```python
from build123d import *

# Parameters (mm, degrees)
F0_R     = 2.725
F1_DEPTH = 10
F2_R     = 1.75
F3_DEPTH = 12.5
F4_R     = 1.8
F4_R_2   = 1.75
F5_DEPTH = 1
F6_R     = 1.75
F7_DEPTH = 4
F9_R     = 1.75


# Not quite as in the source:
# - a fillet or chamfer that OpenCascade refuses, or shapes differently, is made with other operations: its cross-section is extruded or revolved along the edge and cut away or added


with BuildPart() as f1:
    # F0 (on Top) → F1 (new body)
    with BuildSketch(Plane.XY):
        Circle(F0_R)
    extrude(amount=F1_DEPTH)

    # F2 (on face) → F3 (join)
    with BuildSketch(Plane.XY.offset(10)):
        Circle(F2_R)
    extrude(amount=F3_DEPTH)

    # F4 (on face) → F5 (join)
    with BuildSketch(Plane.XY.offset(22.5)):
        Circle(F4_R)
        Circle(F4_R_2, mode=Mode.SUBTRACT)
        Circle(F4_R_2)
    extrude(amount=F5_DEPTH)

    # F6 (on face) → F7 (join)
    with BuildSketch(Plane.XY.offset(23.5)):
        Circle(F6_R)
    extrude(amount=F7_DEPTH)

    # F8: fillet of radius 0.1 on 2 edges, made by hand

    # F8_s1 → F8_t2 (revolve, cut)
    with BuildSketch(Plane.XZ):
        with BuildLine():
            ThreePointArc((1.8, 23.4133974596), (1.7866025404, 23.4633974596), (1.75, 23.5))
            Line((1.75, 23.5), (1.8, 23.5))
            Line((1.8, 23.5), (1.8, 23.4133974596))
        make_face()
    revolve(axis=Axis((0, 0, 23.5), (0, 0, 1)), mode=Mode.SUBTRACT)

    # F8_s3 → F8_t4 (revolve, cut)
    with BuildSketch(Plane.XZ):
        with BuildLine():
            ThreePointArc((1.8, 22.5866025404), (1.7866025404, 22.5366025404), (1.75, 22.5))
            Line((1.75, 22.5), (1.8, 22.5))
            Line((1.8, 22.5), (1.8, 22.5866025404))
        make_face()
    revolve(axis=Axis((0, 0, 22.5), (0, 0, 1)), mode=Mode.SUBTRACT)

    # F9
    f9_edges = [f1.edges().sort_by_distance(p)[0] for p in [
        (-1.75, 0, 27.5),
    ]]
    fillet(f9_edges, radius=F9_R)


solid = f1.part
```
The listing builds one solid part. Answer for the finished solid, in the listing's coordinates (mm). A direction names the side the tool comes from. Give positions to 0.01 mm unless a question says otherwise; leave off trailing zeros. Order: outer loops, then holes, each group sorted by start corner. A loop starts at its lowest first (then second) coordinate and runs counter-clockwise, first axis right, second up. Notation, with made-up numbers: (40, -23) - (98, -23) arc R25 cw to (98, 14) - close; hole circle Ø9 at (63.5, -2). An arc over 180 degrees is marked (long way). Answer in a Markdown table with one row per item. Add a question column.
Q1. Find the intervals of material crossed by line 1 along Z through (x, y) = (-2, 1.55); line 2 along Y through (x, z) = (0.05, 20.25); line 3 along X through (y, z) = (0.3, 21.5), in increasing order. Write a range as [from, to].
Q2. Which of the six approach directions +Z, -Z, +X, -X, +Y, -Y give full straight-line access (tool end or side, diameter ignored) to faces 4 (the cylindrical face through (2.6, 0.82, 4.93)), 5 (the cylindrical face through (1.717, 0.541, 22.994))?
Q3. Given P1, Ø1, axis at y = 1, z = 7, coming from the +X side; P2, Ø3, axis at x = -1.5, z = 20, coming from the -Y side, each flat-ended and moving along its own axis, determine where each tip first touches the part or whether it passes through.
Q4. For a pull along Z with two mould halves and no side action, classify faces 1 (the cylindrical face through (1.617, -0.67, 24.609)), 2 (the flat face through (0, 0, 0)), 3 (the cylindrical face through (1.617, -0.67, 16.163)) as released by +Z, released by -Z, zero draft, split by the parting line, or undercut.
Q5. The part is cut by section A-A (y = 0). Determine the outline of the cut face in (x, z) (3 decimals).
Q6. The part is cut by section D-D (y = -2.05). Determine the outline of the cut face in (x, z).
Q7. The part is cut by section C-C (z = 10.5). Determine the outline of the cut face in (x, y).
Determined:
| question | item | result |
|---|---|---|
| 1 | line 1 | z = [0, 10] |
| 1 | line 2 | y = [-1.75, 1.75] |
| 1 | line 3 | x = [-1.72, 1.72] |
| 2 | face 4 | +Z, -Z |
| 2 | face 5 | +Z |
| 3 | P1 | stops at x = 2.68 |
| 3 | P2 | stops at y = -1.75 |
| 4 | face 1 | zero draft |
| 4 | face 2 | released by -Z |
| 4 | face 3 | undercut |
| 5 | outline | (-2.725, 0) - (2.725, 0) - (2.725, 10) - (1.75, 10) - (1.75, 22.5) arc R0.1 ccw to (1.8, 22.587) - (1.8, 23.413) arc R0.1 ccw to (1.75, 23.5) - (1.75, 25.75) arc R1.75 ccw to (-1.75, 25.75) - (-1.75, 23.5) arc R0.1 ccw to (-1.8, 23.413) - (-1.8, 22.587) arc R0.1 ccw to (-1.75, 22.5) - (-1.75, 10) - (-2.725, 10) - close |
| 6 | outline | (-1.8, 0) - (1.8, 0) - (1.8, 10) - (-1.8, 10) - close |
| 7 | outline | circle Ø3.5 at (0, 0) |
